Autodesk Inventor part; units mm, degrees
ref_plane "YZ Plane" through (0, 0, 0) normal (1, 0, 0) x (0, 1, 0)
ref_plane "XZ Plane" through (0, 0, 0) normal (0, 1, 0) x (-1, 0, 0)
ref_plane "XY Plane" through (0, 0, 0) normal (0, 0, 1) x (1, 0, 0)
sketch "Sketch1" plane through (0, 0, 0) normal (0, 1, 0) x (-1, 0, 0)
  arc A0 (-1.9692, 2.8605) -> (-2.8605, 1.9692) centre (-2.4696, 2.4696) ccw
  line L0 (-2.2319, 1.3405) -> (-2.8605, 1.9692)
  arc A1 (-2.2319, 1.3405) -> (-2.2319, -1.3405) centre (0, 0) ccw
  line L1 (-2.8605, -1.9692) -> (-2.2319, -1.3405)
  arc A2 (-2.8605, -1.9692) -> (-1.9692, -2.8605) centre (-2.4696, -2.4696) ccw
  line L2 (-1.3405, -2.2319) -> (-1.9692, -2.8605)
  arc A3 (-1.3405, -2.2319) -> (1.3405, -2.2319) centre (0, 0) ccw
  line L3 (1.9692, -2.8605) -> (1.3405, -2.2319)
  arc A4 (1.9692, -2.8605) -> (2.8605, -1.9692) centre (2.4696, -2.4696) ccw
  line L4 (2.2319, -1.3405) -> (2.8605, -1.9692)
  arc A5 (2.2319, -1.3405) -> (2.2319, 1.3405) centre (0, 0) ccw
  line L5 (2.8605, 1.9692) -> (2.2319, 1.3405)
  arc A6 (2.8605, 1.9692) -> (1.9692, 2.8605) centre (2.4696, 2.4696) ccw
  line L6 (1.3405, 2.2319) -> (1.9692, 2.8605)
  arc A7 (1.3405, 2.2319) -> (-1.3405, 2.2319) centre (0, 0) ccw
  line L7 (-1.9692, 2.8605) -> (-1.3405, 2.2319)
  arc A8 (-1.6396, -4.5172) -> (-3.8846, -5.4471) centre (-1.6396, -7.6922) ccw
  line L8 (-3.8846, -5.4471) -> (-7.1933, -8.7558)
  arc A9 (-7.1933, -8.7558) -> (-6.4749, -10.4902) centre (-6.4749, -9.4742) ccw
  line L9 (-6.4749, -10.4902) -> (-4.3561, -10.4902)
  arc A10 (-4.3561, -12.7) -> (-4.3561, -10.4902) centre (-4.3561, -11.5951) ccw
  line L10 (-4.3561, -12.7) -> (-10.5918, -12.7)
  arc A11 (-12.7, -10.5918) -> (-10.5918, -12.7) centre (-10.5918, -10.5918) ccw
  line L11 (-12.7, -10.5918) -> (-12.7, -4.3561)
  arc A12 (-10.4902, -4.3561) -> (-12.7, -4.3561) centre (-11.5951, -4.3561) ccw
  line L12 (-10.4902, -4.3561) -> (-10.4902, -6.4749)
  arc A13 (-10.4902, -6.4749) -> (-8.7558, -7.1933) centre (-9.4742, -6.4749) ccw
  line L13 (-8.7558, -7.1933) -> (-5.4471, -3.8846)
  arc A14 (-5.4471, -3.8846) -> (-4.5172, -1.6396) centre (-7.6922, -1.6396) ccw
  line L14 (-4.5172, -1.6396) -> (-4.5172, 1.6396)
  arc A15 (-4.5172, 1.6396) -> (-5.4471, 3.8846) centre (-7.6922, 1.6396) ccw
  line L15 (-5.4471, 3.8846) -> (-8.7558, 7.1933)
  arc A16 (-8.7558, 7.1933) -> (-10.4902, 6.4749) centre (-9.4742, 6.4749) ccw
  line L16 (-10.4902, 6.4749) -> (-10.4902, 4.3561)
  arc A17 (-12.7, 4.3561) -> (-10.4902, 4.3561) centre (-11.5951, 4.3561) ccw
  line L17 (-12.7, 4.3561) -> (-12.7, 10.5918)
  arc A18 (-10.5918, 12.7) -> (-12.7, 10.5918) centre (-10.5918, 10.5918) ccw
  line L18 (-10.5918, 12.7) -> (-4.3561, 12.7)
  arc A19 (-4.3561, 10.4902) -> (-4.3561, 12.7) centre (-4.3561, 11.5951) ccw
  line L19 (-4.3561, 10.4902) -> (-6.4749, 10.4902)
  arc A20 (-6.4749, 10.4902) -> (-7.1933, 8.7558) centre (-6.4749, 9.4742) ccw
  line L20 (-7.1933, 8.7558) -> (-3.8846, 5.4471)
  arc A21 (-3.8846, 5.4471) -> (-1.6396, 4.5172) centre (-1.6396, 7.6922) ccw
  line L21 (-1.6396, 4.5172) -> (1.6396, 4.5172)
  arc A22 (1.6396, 4.5172) -> (3.8846, 5.4471) centre (1.6396, 7.6922) ccw
  line L22 (3.8846, 5.4471) -> (7.1933, 8.7558)
  arc A23 (7.1933, 8.7558) -> (6.4749, 10.4902) centre (6.4749, 9.4742) ccw
  line L23 (6.4749, 10.4902) -> (4.3561, 10.4902)
  arc A24 (4.3561, 12.7) -> (4.3561, 10.4902) centre (4.3561, 11.5951) ccw
  line L24 (4.3561, 12.7) -> (10.5918, 12.7)
  arc A25 (12.7, 10.5918) -> (10.5918, 12.7) centre (10.5918, 10.5918) ccw
  line L25 (12.7, 10.5918) -> (12.7, 4.3561)
  arc A26 (10.4902, 4.3561) -> (12.7, 4.3561) centre (11.5951, 4.3561) ccw
  line L26 (10.4902, 4.3561) -> (10.4902, 6.4749)
  arc A27 (10.4902, 6.4749) -> (8.7558, 7.1933) centre (9.4742, 6.4749) ccw
  line L27 (8.7558, 7.1933) -> (5.4471, 3.8846)
  arc A28 (5.4471, 3.8846) -> (4.5172, 1.6396) centre (7.6922, 1.6396) ccw
  line L28 (4.5172, 1.6396) -> (4.5172, -1.6396)
  arc A29 (4.5172, -1.6396) -> (5.4471, -3.8846) centre (7.6922, -1.6396) ccw
  line L29 (5.4471, -3.8846) -> (8.7558, -7.1933)
  arc A30 (8.7558, -7.1933) -> (10.4902, -6.4749) centre (9.4742, -6.4749) ccw
  line L30 (10.4902, -6.4749) -> (10.4902, -4.3561)
  arc A31 (12.7, -4.3561) -> (10.4902, -4.3561) centre (11.5951, -4.3561) ccw
  line L31 (12.7, -4.3561) -> (12.7, -10.5918)
  arc A32 (10.5918, -12.7) -> (12.7, -10.5918) centre (10.5918, -10.5918) ccw
  line L32 (10.5918, -12.7) -> (4.3561, -12.7)
  arc A33 (4.3561, -10.4902) -> (4.3561, -12.7) centre (4.3561, -11.5951) ccw
  line L33 (4.3561, -10.4902) -> (6.4749, -10.4902)
  arc A34 (6.4749, -10.4902) -> (7.1933, -8.7558) centre (6.4749, -9.4742) ccw
  line L34 (7.1933, -8.7558) -> (3.8846, -5.4471)
  arc A35 (3.8846, -5.4471) -> (1.6396, -4.5172) centre (1.6396, -7.6922) ccw
  line L35 (1.6396, -4.5172) -> (-1.6396, -4.5172)
  dimension "d0" = 1.1049
  dimension "d1" = 2.1082
  dimension "d2" = 1.016
  dimension "d3" = 3.175
  dimension "d4" = 0.635
  dimension "d5" = 2.6035
  dimension "d6" = 2.6035
  dimension "d7" = 2.6035
  dimension "d8" = 2.6035
  dimension "d9" = 45
  dimension "d10" = 45
  dimension "d11" = 45
  dimension "d12" = 45
  dimension "d13" = 45
  dimension "d14" = 45
  dimension "d15" = 45
  dimension "d16" = 90
  dimension "d17" = 90
  dimension "d18" = 45
  dimension "d19" = 45
  dimension "d20" = 90
  dimension "d21" = 90
  dimension "d22" = 90
  dimension "d23" = 90
  dimension "d24" = 90
  dimension "d25" = 90
  dimension "d26" = 8.1828
  dimension "d27" = 17.2172
  dimension "d28" = 23.1902
  dimension "d29" = 25.4
  dimension "d30" = 8.1828
  dimension "d31" = 17.2172
  dimension "d32" = 2.2096
  dimension "d33" = 0.4746
  dimension "d34" = 1.7351
  dimension "d35" = 1.2605
  dimension "d36" = 0.4746
  dimension "d37" = 1.7351
  dimension "d38" = 12.7
  dimension "d39" = 12.7
  dimension "d40" = 10.4902
  dimension "d41" = 12.7
  dimension "d42" = 1.1048
  dimension "d43" = 1.1048
  dimension "d44" = 1.1048
  dimension "d45" = 0.6303
  dimension "d46" = 0.6303
  dimension "d47" = 0.6303
  dimension "d48" = 0.6303
  dimension "d49" = 0.6303
  dimension "d50" = 10.4902
  dimension "d51" = 10.4902
  dimension "d52" = 1.1048
  dimension "d53" = 1.1048
  dimension "d54" = 12.7
  dimension "d55" = 12.7
  dimension "d56" = 10.4902
  dimension "d57" = 12.7
  dimension "d58" = 8.3439
  dimension "d59" = 17.0561
  dimension "d60" = 8.3439
  dimension "d61" = 8.3439
  dimension "d62" = 9.8395
  dimension "d63" = 9.8395
extrude "Extrusion1" add sketch "Sketch1" along normal mid plane 25.4
properties part number "1010-S-BLACK-FB" material "6061-T6"
Source: CAD feature listing. Evaluate the final solid. Frame: model axes, mm. A direction names the side the tool comes from. Round coordinates to 2 decimals unless told otherwise and drop trailing zeros. Loops run counter-clockwise (first coordinate to the right, second up) from the corner with the lowest first, then second, coordinate; pieces in that order, holes last. Notation, with made-up numbers: M -0.75,-7 L 20.25,-7 A14 cw 20.25,16 Z; hole C -2.5,-1.75 d4. An arc over 180 degrees is marked long. Use a Markdown table: item, result. Add a question column.
1. Contact query for flat-ended pins moving along their axis: pin 1 (3.5 mm diameter, centred on y = 6, z = 0, fed in from +X); pin 2 (1.6 mm diameter, centred on x = 0, y = 4, fed in from -Z); pin 3 (0.8 mm diameter, centred on x = -2.47, z = -2.47, fed in from -Y); pin 4 (3.5 mm diameter, centred on x = 0.5, y = 1, fed in from +Z). Output: stop coordinate, or through.
2. Ray query, line 1 along Z through (x, y) = (-6.75, -7); line 2 along X through (y, z) = (2.5, 5.5); line 3 along Z through (x, y) = (3.5, 6). Return the intervals inside material, ascending. Write a range as [from, to].
3. Cut plane B-B, the plane z = 9.5. Output: boundary loops of the cut face in (x, y), and give its area (3 significant figures).
4. Cut plane A-A, the plane x = 0. Output: boundary loops of the cut face in (y, z).
5. Pull-direction query (Z, two-part tool) for faces 3 (the flat face through (-4.517, 0, 0)), 4 (the flat face through (-12.7, 0, -7)), 5 (the flat face through (0, 0, -4.517)); classes: +Z half, -Z half, draft (parallel to the pull), parting line (faces both ways), or undercut.
6. Set-up query: faces 1 (the cylindrical face through (12.066, -0.178, -12.099)), 2 (the cylindrical face through (11.57, -0.18, 3.25)). Return all of +Z, -Z, +X, -X, +Y, -Y with unobstructed straight access to the full face (end or side cutting, diameter ignored); none if empty.
Solution:
| question | item | result |
|---|---|---|
| 1 | pin 1 | stops at x = 4.52 |
| 1 | pin 2 | stops at z = -4.52 |
| 1 | pin 3 | passes through |
| 1 | pin 4 | stops at z = 4.58 |
| 2 | line 1 | z = [-12.7, -10.45], [-8.31, -5.19], [5.19, 8.31], [10.45, 12.7] |
| 2 | line 2 | x = [-12.7, -10.49], [-7.06, -3.94], [3.94, 7.06], [10.49, 12.7] |
| 2 | line 3 | z = [-12.29, -10.9], [-5.12, 5.12], [10.9, 12.29] |
| 3 | outline | M -12.7,-12.7 L -7.49,-12.7 L -7.49,12.7 L -12.7,12.7 Z; M 7.49,-12.7 L 12.7,-12.7 L 12.7,12.7 L 7.49,12.7 Z |
| 3 | area | 265 mm2 |
| 4 | outline | M -12.7,-4.52 L 12.7,-4.52 L 12.7,-2.6 L -12.7,-2.6 Z; M -12.7,2.6 L 12.7,2.6 L 12.7,4.52 L -12.7,4.52 Z |
| 5 | face 3 | undercut |
| 5 | face 4 | draft |
| 5 | face 5 | -Z half |
| 6 | face 1 | -Z, +X, +Y, -Y |
| 6 | face 2 | +Y, -Y |
